The model under review builds one solid part; all positions refer to its coordinate system, in mm. Face numbers are marked on the shaded views. A direction names the side the tool comes from. Give positions to 0.01 mm unless a question says otherwise; leave off trailing zeros. Order: outer loops, then holes, each group sorted by start corner. A loop starts at its lowest first (then second) coordinate and runs counter-clockwise, first axis right, second up. Notation, with made-up numbers: (-12, 12.25) -> (41, 12.25) arc R34 cw to (41, 43.25) -> close; hole circle Ø5 at (-6.75, 12). An arc over 180 degrees is marked (long way). Use one line per item in the form item = value.
```python
from build123d import *

# Parameters (mm, degrees)
F2_R     = 1
F3_DEPTH = 4
F4_R     = 1
F5_DEPTH = 3


with BuildPart() as f1:
    # F0 (on Front) → F1 (revolve)
    with BuildSketch(Plane.XZ):
        Polygon((1, 22), (0, 22), (0, 0), (0, -1.8), (1, -1.8), (1, 0), (9.5, 0), (11.5, 2), (11.5, 3), (11, 3), (11, 3.5), (11.5, 3.5), (11.5, 4.5), (9.5, 4.5), (9.5, 4.8), (11.5, 4.8), (11.5, 14.5), (7.5, 18.5), (1, 18.5), align=None)
        Polygon((2, 16.5), (2, 17.5), (7.085786, 17.5), (10.5, 14.085786), (10.5, 10.695516), (1, 10.695516), (1, 16.5), align=None, mode=Mode.SUBTRACT)
    revolve(axis=Axis((0, 0, 11), (0, 0, -1)))

    # F2 (on face) → F3 (cut)
    with BuildSketch(Plane.XY.offset(18.5)):
        with Locations((4.5, 0)):
            Circle(F2_R)
        with Locations((0, 4.5)):
            Circle(F2_R)
        with Locations((-4.5, 0)):
            Circle(F2_R)
        with Locations((0, -4.5)):
            Circle(F2_R)
        with BuildLine():
            Line((-8.947627, -2.999543), (-9.052373, -2.999543))
            ThreePointArc((-9.052373, -2.999543), (-9, -3), (-8.947627, -2.999543))
        make_face()
        with BuildLine():
            Line((-15.532091, -2.999543), (-9.052373, -2.999543))
            Line((-9.052373, -2.999543), (-8.947627, -2.999543))
            ThreePointArc((-8.947627, -2.999543), (-6, 0), (-8.947627, 2.999543))
            Line((-8.947627, 2.999543), (-9.052373, 2.999543))
            Line((-9.052373, 2.999543), (-15.532091, 2.999543))
            Line((-15.532091, 2.999543), (-15.532091, -2.999543))
        make_face()
        with BuildLine():
            Line((-9.052373, 2.999543), (-8.947627, 2.999543))
            ThreePointArc((-8.947627, 2.999543), (-9, 3), (-9.052373, 2.999543))
        make_face()
        with BuildLine():
            Line((-10.363726, -11.951414), (-5.168365, -14.950957))
            Line((-5.168365, -14.950957), (-1.928506, -9.339356))
            Line((-1.928506, -9.339356), (-1.876133, -9.248644))
            ThreePointArc((-1.876133, -9.248644), (-3, -5.196152), (-7.071494, -6.249101))
            Line((-7.071494, -6.249101), (-7.123867, -6.339813))
            Line((-7.123867, -6.339813), (-10.363726, -11.951414))
        make_face()
        with BuildLine():
            Line((-1.876133, -9.248644), (-1.928506, -9.339356))
            ThreePointArc((-1.928506, -9.339356), (-1.901924, -9.294229), (-1.876133, -9.248644))
        make_face()
        with BuildLine():
            ThreePointArc((-7.071494, -6.249101), (-7.098076, -6.294229), (-7.123867, -6.339813))
            Line((-7.123867, -6.339813), (-7.071494, -6.249101))
        make_face()
        with BuildLine():
            Line((5.168365, -14.950957), (10.363726, -11.951414))
            Line((10.363726, -11.951414), (7.123867, -6.339813))
            Line((7.123867, -6.339813), (7.071494, -6.249101))
            ThreePointArc((7.071494, -6.249101), (3, -5.196152), (1.876133, -9.248644))
            Line((1.876133, -9.248644), (1.928506, -9.339356))
            Line((1.928506, -9.339356), (5.168365, -14.950957))
        make_face()
        with BuildLine():
            Line((7.071494, -6.249101), (7.123867, -6.339813))
            ThreePointArc((7.123867, -6.339813), (7.098076, -6.294229), (7.071494, -6.249101))
        make_face()
        with BuildLine():
            ThreePointArc((1.876133, -9.248644), (1.901924, -9.294229), (1.928506, -9.339356))
            Line((1.928506, -9.339356), (1.876133, -9.248644))
        make_face()
        with BuildLine():
            Line((15.532091, -2.999543), (15.532091, 2.999543))
            Line((15.532091, 2.999543), (9.052373, 2.999543))
            Line((9.052373, 2.999543), (8.947627, 2.999543))
            ThreePointArc((8.947627, 2.999543), (6, 0), (8.947627, -2.999543))
            Line((8.947627, -2.999543), (9.052373, -2.999543))
            Line((9.052373, -2.999543), (15.532091, -2.999543))
        make_face()
        with BuildLine():
            Line((8.947627, 2.999543), (9.052373, 2.999543))
            ThreePointArc((9.052373, 2.999543), (9, 3), (8.947627, 2.999543))
        make_face()
        with BuildLine():
            ThreePointArc((8.947627, -2.999543), (9, -3), (9.052373, -2.999543))
            Line((9.052373, -2.999543), (8.947627, -2.999543))
        make_face()
        with BuildLine():
            Line((10.363726, 11.951414), (5.168365, 14.950957))
            Line((5.168365, 14.950957), (1.928506, 9.339356))
            Line((1.928506, 9.339356), (1.876133, 9.248644))
            ThreePointArc((1.876133, 9.248644), (3, 5.196152), (7.071494, 6.249101))
            Line((7.071494, 6.249101), (7.123867, 6.339813))
            Line((7.123867, 6.339813), (10.363726, 11.951414))
        make_face()
        with BuildLine():
            Line((1.876133, 9.248644), (1.928506, 9.339356))
            ThreePointArc((1.928506, 9.339356), (1.901924, 9.294229), (1.876133, 9.248644))
        make_face()
        with BuildLine():
            ThreePointArc((7.071494, 6.249101), (7.098076, 6.294229), (7.123867, 6.339813))
            Line((7.123867, 6.339813), (7.071494, 6.249101))
        make_face()
        with BuildLine():
            Line((-5.168365, 14.950957), (-10.363726, 11.951414))
            Line((-10.363726, 11.951414), (-7.123867, 6.339813))
            Line((-7.123867, 6.339813), (-7.071494, 6.249101))
            ThreePointArc((-7.071494, 6.249101), (-3, 5.196152), (-1.876133, 9.248644))
            Line((-1.876133, 9.248644), (-1.928506, 9.339356))
            Line((-1.928506, 9.339356), (-5.168365, 14.950957))
        make_face()
        with BuildLine():
            Line((-7.071494, 6.249101), (-7.123867, 6.339813))
            ThreePointArc((-7.123867, 6.339813), (-7.098076, 6.294229), (-7.071494, 6.249101))
        make_face()
        with BuildLine():
            ThreePointArc((-1.876133, 9.248644), (-1.901924, 9.294229), (-1.928506, 9.339356))
            Line((-1.928506, 9.339356), (-1.876133, 9.248644))
        make_face()
    extrude(amount=-F3_DEPTH, mode=Mode.SUBTRACT)

    # F4 (on face) → F5 (cut)
    with BuildSketch(Plane(origin=(0, 0, 0), x_dir=(1, 0, 0), z_dir=(0, 0, -1))):
        with Locations((6, 0)):
            Circle(F4_R)
        with Locations((-6, 0)):
            Circle(F4_R)
        with Locations((0, -8)):
            Circle(F4_R)
        with Locations((0, 8)):
            Circle(F4_R)
    extrude(amount=-F5_DEPTH, mode=Mode.SUBTRACT)


solid = f1.part
```
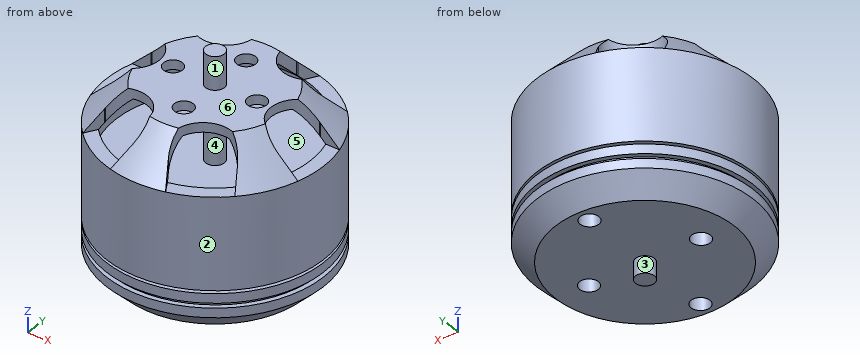
1. For L1, parallel to Y at x = 0, z = 13.2; L2, parallel to X at y = 0, z = 2.05; L3, parallel to Z at x = 1.5, y = 2, list the stretches that pass through material, from the lowest coordinate up.
Values:
L1 = -11.5 to -10.5, -1 to 1, 10.5 to 11.5
L2 = -11.5 to -7, -5 to 5, 7 to 11.5
L3 = 0 to 10.7, 17.5 to 18.5
2. Tool access review of the marked faces 1 and 2: name each direction out of +Z, -Z, +X, -X, +Y, -Y from which nothing blocks a thin tool from reaching the whole face with its end or side.
Values:
face_1 = +Z
face_2 = +Z, -Z
3. Add section B-B on z = 5.25. Give the boundary of the cut face in (x, y).
Values:
outline = circle Ø23 at (0, 0)
4. The part is to be moulded in two halves that separate along Y. For the marked faces 3, 4, 5 and 6, say which applies: +Y half, -Y half, draft (parallel to the pull), parting line (faces both ways), or undercut.
Values:
face_3 = parting line
face_4 = undercut
face_5 = undercut
face_6 = draft
5. For pin 1 Ø1.3 at (x, y) = (-4.5, -10) entering from +Z; pin 2 Ø1 at (x, z) = (-6.5, 12.5) entering from +Y; pin 3 Ø3 at (x, y) = (-2.5, 4) entering from +Z, all flat-tipped, find the tip position at first contact; note any pin that passes through.
Values:
pin_1 = 14.5
pin_2 = 9.81
pin_3 = 18.5
6. Add section A-A on z = 0.5. Give the boundary of the cut face in (x, y).
Values:
outline = circle Ø20 at (0, 0); hole circle Ø2 at (-6, 0); hole circle Ø2 at (0, -8); hole circle Ø2 at (0, 8); hole circle Ø2 at (6, 0)
